Geometry check sheet. Reference: the model listing, model coordinates, mm. A direction names the side the tool comes from. Coordinates: 2 decimals unless noted, no trailing zeros. Write each loop counter-clockwise with the first axis right and the second up, starting at its lowest first coordinate (ties: lowest second). Pieces come first, ordered by that corner, then holes. Notation, with made-up numbers: (27.25, -38.75) -> (59.25, -38.75) arc R31 ccw to (59.25, -9.75) -> close; hole circle Ø2 at (16.5, 38.5). An arc over 180 degrees is marked (long way). Answer as CSV lines item,"result".
```python
from build123d import *

# Parameters (mm, degrees)
CROQUIS1_W                 = 20
CROQUIS1_H                 = 40
SALIENTE_EXTRUIR1_DEPTH    = 30
CROQUIS2_W                 = 20
CROQUIS2_H                 = 40
CROQUIS2_W_2               = 18
CROQUIS2_H_2               = 38
CORTAR_EXTRUIR1_DEPTH      = 10
CORTAR_EXTRUIR2_DEPTH      = 41.755367745
CORTAR_EXTRUIR2_DEPTH_BACK = 41.755367745
CROQUIS4_R                 = 3
SALIENTE_EXTRUIR2_DEPTH    = 1


with BuildPart() as part:
    # Croquis1 → Saliente-Extruir1 (new body)
    with BuildSketch(Plane(origin=(0, 0, 0), x_dir=(1, 0, 0), z_dir=(0, 1, 0))):
        Rectangle(CROQUIS1_W, CROQUIS1_H)
    extrude(amount=SALIENTE_EXTRUIR1_DEPTH)

    # Croquis2 → Cortar-Extruir1 (cut)
    with BuildSketch(Plane(origin=(0, 30, 0), x_dir=(1, 0, 0), z_dir=(0, 1, 0))):
        Rectangle(CROQUIS2_W, CROQUIS2_H)
        Rectangle(CROQUIS2_W_2, CROQUIS2_H_2, mode=Mode.SUBTRACT)
    extrude(amount=-CORTAR_EXTRUIR1_DEPTH, mode=Mode.SUBTRACT)

    # Croquis3 → Cortar-Extruir2 (cut, two sides: drawn at the far end of the back side and taken through both)
    with BuildSketch(Plane.ZY.offset(9).offset(-CORTAR_EXTRUIR2_DEPTH_BACK)):
        with BuildLine():
            Line((19, 30), (-10.226390802, 30))
            add(Edge.make_bspline(
                [(-10.226390802, 30), (5.11136514, 23.592400747), (19, 30)],
                knots=[0, 0, 0, 1, 1, 1], degree=2))
        make_face()
    extrude(amount=CORTAR_EXTRUIR2_DEPTH + CORTAR_EXTRUIR2_DEPTH_BACK, mode=Mode.SUBTRACT)

    # Croquis4 → Saliente-Extruir2 (add)
    with BuildSketch(Plane(origin=(0, 30, 0), x_dir=(1, 0, 0), z_dir=(0, 1, 0))):
        with Locations(Location((0, 14.613195401, 0), (0, 0, 90))):
            Circle(CROQUIS4_R)
    extrude(amount=SALIENTE_EXTRUIR2_DEPTH)


solid = part.part
```
Item 1: Set-up check for faces 1 (the flat face through (0, 25, 19)), 2 (the flat face through (0, 25, -19)), 3 (the flat face through (-9, 24, 0)), 4 (the flat face through (9, 24, 0)): record each of +Z, -Z, +X, -X, +Y, -Y from which the full face is reachable in a straight line by a thin tool's end or side.
Responses:
face 1,"+Z, +X, -X, +Y"
face 2,"-Z, +X, -X, +Y"
face 3,"+Z, -Z, -X, +Y"
face 4,"+Z, -Z, +X, +Y"
Item 2: Depth check by flat-ended pin: pin 1 Ø5 at (y, z) = (23, -0.5) entering from -X; pin 2 Ø3 at (x, y) = (-2.5, 26.5) entering from +Z; pin 3 Ø3 at (x, y) = (1.5, 26) entering from -Z. Enter the tip coordinate at first touch or a pass-through.
Responses:
pin 1,"stops at x = -9"
pin 2,"stops at z = 19"
pin 3,"stops at z = -19"
Item 3: Cross-section at A-A, the plane y = 21. Record the cut outline in (x, z), plus the area to 3 significant figures.
Responses:
outline,"(-9, -19) -> (9, -19) -> (9, 19) -> (-9, 19) -> close"
area,"684 mm2"
Item 4: Thickness scan on probe 1 along Y at (x, z) = (-3.5, -12); probe 2 along X at (y, z) = (29, -17.5); probe 3 along Z at (x, y) = (-7.5, 20.5). Record the ranges inside material, lowest first.
Responses:
probe 1,"y = 0 to 30"
probe 2,"x = -9 to 9"
probe 3,"z = -19 to 19"
